Model file for the job. Use its own axes, mm. Round coordinates to 2 decimals unless told otherwise and drop trailing zeros. Order: outer loops, then holes, each group sorted by start corner. A loop starts at its lowest first (then second) coordinate and runs counter-clockwise, first axis right, second up. Notation, with made-up numbers: (84, -9) -> (88, -9) arc R17 cw to (88, 11) -> close; hole circle Ø1 at (-2.5, -24.5). An arc over 180 degrees is marked (long way). Put each result on its own line as item: value. Start each with the question number.
Q1. Cut at B-B, the plane x = 0. List the corners of the cut face in (y, z).
Q2. Cut at D-D, the plane x = -6. List the corners of the cut face in (y, z).
Q3. Cut at A-A, the plane y = 20. List the corners of the cut face in (x, z), and give its area (3 significant figures).
Q4. Cut at C-C, the plane z = 0.95. List the corners of the cut face in (x, y), and give its area (3 significant figures).
Q5. Probe L1, parallel to Y at x = 0, z = 1.1; L2, parallel to X at y = -1, z = 1.25; L3, parallel to X at y = -3, z = 1.15. List the from-to ranges inside material, lowest first.
Q6. Flat gauge pin, fed straight in: P1, Ø13.5, axis at x = 0, y = 0, coming from the +Z side. Where does the tip first touch, or does it go through?
from build123d import *

# Parameters (mm, degrees)
SKETCH_1_R          = 1.55
EXTRUDE_1_DEPTH     = 1.5
SKETCH_2_R          = 11.05
CUT_EXTRUDE_1_DEPTH = 1.5


with BuildPart() as part:
    # 草图1 → 凸台-拉伸1 (new body)
    with BuildSketch(Plane.XY):
        with BuildLine():
            Line((-2.598076211, 21.5), (-19.918584287, -8.5))
            ThreePointArc((-19.918584287, -8.5), (-19.918584287, -11.5), (-17.320508076, -13))
            Line((-17.320508076, -13), (17.320508076, -13))
            ThreePointArc((17.320508076, -13), (19.918584287, -11.5), (19.918584287, -8.5))
            Line((19.918584287, -8.5), (2.598076211, 21.5))
            ThreePointArc((2.598076211, 21.5), (0, 23), (-2.598076211, 21.5))
        make_face()
        with Locations((0, 20)):
            Circle(SKETCH_1_R, mode=Mode.SUBTRACT)
        with Locations((-17.320508076, -10)):
            Circle(SKETCH_1_R, mode=Mode.SUBTRACT)
        with Locations((17.320508076, -10)):
            Circle(SKETCH_1_R, mode=Mode.SUBTRACT)
    extrude(amount=EXTRUDE_1_DEPTH)

    # 草图2 → 切除-拉伸1 (cut)
    with BuildSketch(Plane.XY.offset(1.5)):
        Circle(SKETCH_2_R)
    extrude(amount=-CUT_EXTRUDE_1_DEPTH, mode=Mode.SUBTRACT)


solid = part.part
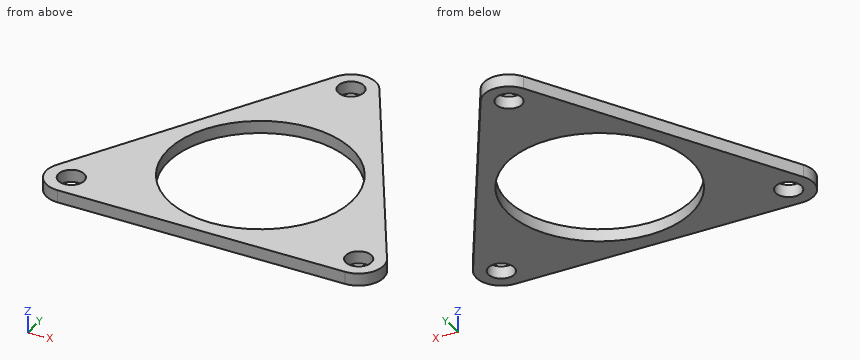
Ans:
1. outline: (-13, 0) -> (-11.05, 0) -> (-11.05, 1.5) -> (-13, 1.5) -> close; (11.05, 0) -> (18.45, 0) -> (18.45, 1.5) -> (11.05, 1.5) -> close; (21.55, 0) -> (23, 0) -> (23, 1.5) -> (21.55, 1.5) -> close
2. outline: (-13, 0) -> (-9.28, 0) -> (-9.28, 1.5) -> (-13, 1.5) -> close; (9.28, 0) -> (15.61, 0) -> (15.61, 1.5) -> (9.28, 1.5) -> close
3. outline: (-3.46, 0) -> (-1.55, 0) -> (-1.55, 1.5) -> (-3.46, 1.5) -> close; (1.55, 0) -> (3.46, 0) -> (3.46, 1.5) -> (1.55, 1.5) -> close
3. area: 5.74 mm^2
4. outline: (-19.92, -8.5) arc R3 ccw to (-17.32, -13) -> (17.32, -13) arc R3 ccw to (19.92, -8.5) -> (2.6, 21.5) arc R3 ccw to (-2.6, 21.5) -> close; hole circle Ø3.1 at (-17.32, -10); hole circle Ø22.1 at (0, 0); hole circle Ø3.1 at (0, 20); hole circle Ø3.1 at (17.32, -10)
4. area: 453 mm^2
5. L1: y = -13 to -11.05, 11.05 to 18.45, 21.55 to 23
5. L2: x = -15.59 to -11, 11 to 15.59
5. L3: x = -16.74 to -10.63, 10.63 to 16.74
6. P1: passes through
